```python
from build123d import *

# Parameters (mm, degrees)
F2_R     = 30
F2_R_2   = 15
F3_DEPTH = 2
F4_SIZE  = 1.99999
F5_R     = 4.5
F6_DEPTH = 25
F7_COUNT = 4
F8_W     = 7.5
F8_H     = 7.5
F9_DEPTH = 50


# Not quite as in the source:
# - a fillet or chamfer is up to 0.001 mm smaller than in the source, because OpenCascade refuses the exact size


with BuildPart() as f1:
    # F0 (on Right) → F1 (revolve)
    with BuildSketch(Plane.YZ):
        Polygon((0, 15), (0, 64.5), (-24, 64.5), (-24, 60.9), (-15, 59.7), (-15, 30), (-36, 30), (-36, 15), align=None)
    revolve(axis=Axis((0, -28.2661654055, 0), (0, -1, 0)))

    # F2 (on face) → F3 (join)
    with BuildSketch(Plane(origin=(0, 0, 0), x_dir=(-1, 0, 0), z_dir=(0, 1, 0))):
        Circle(F2_R)
        Circle(F2_R_2, mode=Mode.SUBTRACT)
    extrude(amount=F3_DEPTH)

    # F4 (size 2 in the source; OpenCascade refuses exactly that, so slightly less here)
    f4_edges = [f1.edges().sort_by_distance(p)[0] for p in [
        (30, 2, 0),
    ]]
    chamfer(f4_edges, length=F4_SIZE)

    # F5 (on face) → F6 (cut)
    with BuildSketch(Plane(origin=(0, 0, 0), x_dir=(-1, 0, 0), z_dir=(0, 1, 0))):
        with Locations((0, 45)):
            Circle(F5_R)
    f6 = extrude(amount=-F6_DEPTH, mode=Mode.SUBTRACT)

    # F7: F6 ×4 about axis
    f7_axis = Axis((0, 2, 0), (0, 1, 0))
    for i in range(1, F7_COUNT):
        add(f6.rotate(f7_axis, i * 360 / F7_COUNT), mode=Mode.SUBTRACT)

    # F8 (on face) → F9 (cut)
    with BuildSketch(Plane(origin=(0, 2, 0), x_dir=(-1, 0, 0), z_dir=(0, 1, 0))):
        with Locations((0, 15)):
            Rectangle(F8_W, F8_H)
    extrude(amount=-F9_DEPTH, mode=Mode.SUBTRACT)


solid = f1.part
```
Source: CAD feature listing. Evaluate the final solid. Frame: model axes, mm. A direction names the side the tool comes from. Round coordinates to 2 decimals unless told otherwise and drop trailing zeros. Write each loop counter-clockwise with the first axis right and the second up, starting at its lowest first coordinate (ties: lowest second). Pieces come first, ordered by that corner, then holes. Notation, with made-up numbers: M 39.25,42.25 L 63.25,42.25 A6 ccw 63.25,46.25 Z; hole C 40,40.25 d10. An arc over 180 degrees is marked long. Answer as a JSON object with one key per item and string values. Group by question number.
(1) Section query D-D on y = -28. Output: boundary loops of the cut face in (x, z), then the cut area to 3 significant figures.
(2) Section query A-A on x = 0. State how many separate pieces and enclosed holes the cut face has, then the cut area to 3 significant figures.
(3) Mould query, pull axis X, two halves, no side actions, for faces 5 (the flat face through (-12, 2, -12)), 6 (the cylindrical face through (0.98, -7.4, 40.61)), 7 (the cylindrical face through (-19.374, -12.168, 61.522)). Classes: +X half, -X half, draft (parallel to the pull), parting line (faces both ways), or undercut.
(4) Ray query, line 1 (X direction, y = -11, z = 0); line 2 (Z direction, x = 0, y = -9.75); line 3 (Z direction, x = 0.5, y = -30.5). Return the intervals inside material, ascending. Write a range as [from, to].
(5) Section query C-C on y = -8. Output: boundary loops of the cut face in (x, z).
(6) Reachability of faces 1 (the flat face through (-3.75, -17, 17)), 2 (the flat face through (47, -24, -39)), 3 (the flat face through (13, 0, -28)), 4 (the flat face through (-14, -36, 6)) from +Z, -Z, +X, -X, +Y, -Y: full face, straight path, thin tool, end or side. Return the list, or none.
(7) First-contact query: pin 1 (5 mm diameter, centred on x = -38.5, z = -26.5, fed in from -Y); pin 2 (3 mm diameter, centred on y = -6, z = 48.5, fed in from +X); pin 3 (5 mm diameter, centred on x = 22, y = -20.5, fed in from -Z). Flat tips, straight axial feed; report the tip coordinate or a pass-through.
Computed values:
{
 "1": {"outline": "C 0,0 d60; hole M -3.75,14.52 A15 ccw long 3.75,14.52 L 3.75,18.75 L -3.75,18.75 Z", "area": "2,090 mm^2"},
 "2": {"separate pieces": "4", "enclosed holes": "0", "area": "1,830 mm^2"},
 "3": {"face 5": "draft", "face 6": "undercut", "face 7": "parting line"},
 "4": {"line 1": "[-64.5, -49.5], [-40.5, -15], [15, 40.5], [49.5, 64.5]", "line 2": "[-64.5, -49.5], [-40.5, -15], [18.75, 40.5], [49.5, 64.5]", "line 3": "[-30, -14.99], [18.75, 30]"},
 "5": {"outline": "C 0,0 d129; hole C -45,0 d9; hole C 0,-45 d9; hole C 0,45 d9; hole M -3.75,14.52 A15 ccw long 3.75,14.52 L 3.75,18.75 L -3.75,18.75 Z; hole C 45,0 d9"},
 "6": {"face 1": "+Y, -Y", "face 2": "-Y", "face 3": "+Y", "face 4": "+Z, -Z, +X, -X, -Y"},
 "7": {"pin 1": "y = -15", "pin 2": "x = 44.17", "pin 3": "z = -61.48"}
}
